Job drawing, mm, ordinate dimensions from the low corner. One solid piece. Round coordinates to 2 decimals unless told otherwise and drop trailing zeros. Write each loop counter-clockwise with the first axis right and the second up, starting at its lowest first coordinate (ties: lowest second). Pieces come first, ordered by that corner, then holes. Notation, with made-up numbers: (25.25, 42) - (66.25, 42) arc R16 cw to (66.25, 60) - close; hole circle Ø8 at (41.5, -4). An arc over 180 degrees is marked (long way). Write each question's results on one line, items separated by ' | '.
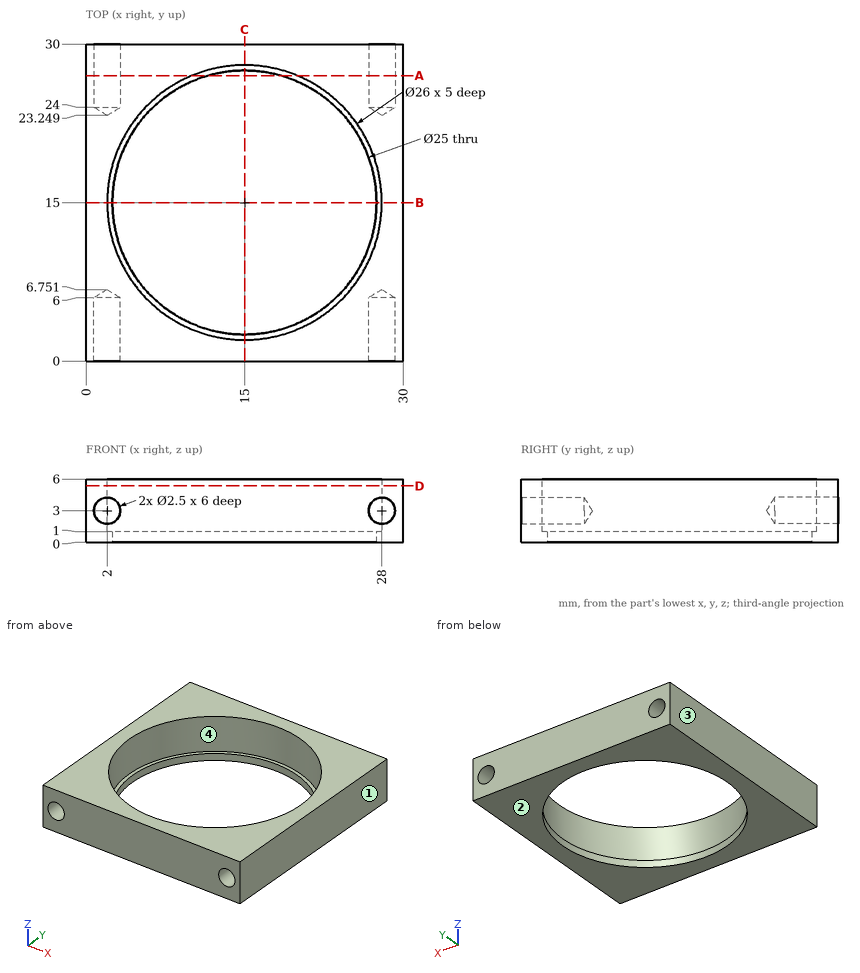
(1) Slice it at D-D, the plane z = 5.35. Write the cut outline in (x, y), and give its area (3 significant figures).
Worked answers:
outline: (0, 0) - (30, 0) - (30, 30) - (0, 30) - close; hole circle Ø26 at (15, 15) | area: 369 mm2
(2) Flat gauge pins, fed straight in: pin 1 Ø1.5 at (x, z) = (28, 3) entering from +Y; pin 2 Ø2 at (x, z) = (28, 3) entering from -Y; pin 3 Ø15 at (x, y) = (15, 15) entering from +Z; pin 4 Ø1.5 at (x, z) = (2, 3) entering from -Y. Where does each tip first touch, or does it go through?
Worked answers:
pin 1: stops at y = 23.7 | pin 2: stops at y = 6.15 | pin 3: passes through | pin 4: stops at y = 6.3
(3) Drill centre lines: probe 1 along Y at (x, z) = (15, 2.6); probe 2 along Y at (x, z) = (15, 0.6); probe 3 along Z at (x, y) = (2, 25.4). Where is each one in solid material? Low to high. Write a range as [from, to].
Worked answers:
probe 1: y = [0, 2], [28, 30] | probe 2: y = [0, 2.5], [27.5, 30] | probe 3: z = [0, 1.75], [4.25, 6]
(4) Two-plate mould, pull along X, no slides. Class the marked faces 1, 2, 3 and 4: released by +X, released by -X, zero draft, split by the parting line, or undercut.
Worked answers:
face 1: released by +X | face 2: zero draft | face 3: released by -X | face 4: undercut
(5) Slice it at A-A, the plane y = 27. Write the cut outline in (x, z).
Worked answers:
outline: (0, 0) - (11.5, 0) - (11.5, 1) - (10, 1) - (10, 6) - (0, 6) - close; (18.5, 0) - (30, 0) - (30, 6) - (20, 6) - (20, 1) - (18.5, 1) - close; hole circle Ø2.5 at (2, 3); hole circle Ø2.5 at (28, 3)
(6) Slice it at B-B, the plane y = 15. Write the cut outline in (x, z).
Worked answers:
outline: (0, 0) - (2.5, 0) - (2.5, 1) - (2, 1) - (2, 6) - (0, 6) - close; (27.5, 0) - (30, 0) - (30, 6) - (28, 6) - (28, 1) - (27.5, 1) - close
